Autodesk Inventor part; units mm, degrees
ref_plane "YZ Plane" through (0, 0, 0) normal (1, 0, 0) x (0, 1, 0)
ref_plane "XZ Plane" through (0, 0, 0) normal (0, 1, 0) x (-1, 0, 0)
ref_plane "XY Plane" through (0, 0, 0) normal (0, 0, 1) x (1, 0, 0)
sketch "Sketch1" plane through (0, 0, 0) normal (1, 0, 0) x (0, 1, 0)
  line L0 (0, 0) -> (55, 0)
  line L1 (55, 0) -> (55, -242)
  line L2 (55, -242) -> (0, -242)
  line L3 (0, -242) -> (0, 0)
  dimension "d0" = 55
  dimension "d1" = 242
extrude "Extrusion1" add sketch "Sketch1" along normal blind 355
sketch "Sketch3" plane through (0, 55, 0) normal (0, 1, 0) x (1, 0, 0)
  circle A0 centre (200, 120) radius 10
  point P0 (0, 0)
  point P1 (0, 0)
  dimension "d8" = 20
extrude "Extrusion3" cut sketch "Sketch3" against normal through all
sketch "Sketch4" plane through (0, 55, 0) normal (0, 1, 0) x (1, 0, 0)
  line L0 (15, 15) -> (340, 15)
  line L1 (340, 15) -> (340, 227)
  line L2 (340, 227) -> (15, 227)
  line L3 (15, 227) -> (15, 15)
  line L4 (355, 242) -> (355, 0)
  line L5 (0, 242) -> (355, 242)
  point P0 (0, 0)
  point P1 (0, 0)
  dimension "d11" = 15
  dimension "d12" = 15
extrude "Extrusion4" cut sketch "Sketch4" against normal blind 35
sketch "Sketch5" plane through (0, 0, 0) normal (0, 0, 1) x (1, 0, 0)
  circle A0 centre (161.4027, 23.0942) radius 3
  line L0 (0, 55) -> (0, 0)
  line L1 (355, 55) -> (355, 0)
  line L2 (0, 0) -> (355, 0)
  dimension "d15" = 6
  dimension "d18" = 161.4027
  dimension "d19" = 355
  dimension "d20" = 23.0942
extrude "Extrusion5" cut sketch "Sketch5" against normal through all
ref_plane "Work Plane1" through (0, 0, -121) normal (0, 0, -1) x (-1, 0, 0)
properties part number "basefresh" material "Wood (Cherry)"
Check sheet for the modelled part. Datum: model origin and axes. Units: mm. A direction names the side the tool comes from. Round coordinates to 2 decimals unless told otherwise and drop trailing zeros. Loops run counter-clockwise (first coordinate to the right, second up) from the corner with the lowest first, then second, coordinate; pieces in that order, holes last. Notation, with made-up numbers: (18.5, -28) - (41.5, -28) arc R36 ccw to (41.5, 7) - close; hole circle Ø9 at (73.25, 46). An arc over 180 degrees is marked (long way). Write item = value, one per line. Start each with the question number.
Q1. Section check D-D (z = -51.5). Record the boundary of the cut face in (x, y), plus the area to 3 significant figures.
Q2. Section check A-A (x = 200). Record the boundary of the cut face in (y, z), plus the area to 3 significant figures.
Q3. Thickness scan on L1, parallel to X at y = 24, z = -116; L2, parallel to Z at x = 200, y = 5.75; L3, parallel to Z at x = 302, y = 27.5. Record the ranges inside material, lowest first.
Q4. Release check for a two-part mould opening along Z. For faces 3 (the face through (205.38, 10.14, -128.43)), 4 (the face through (164, 55, -13)), 5 (the face through (175, 38, -15)), 6 (the face through (175, 28, -242)) record: pulls with the +Z half, pulls with the -Z half, needs draft (parallel to the pull), parting line crosses it, or undercut.
Q5. Section check B-B (z = -120). Record the boundary of the cut face in (x, y), plus the area to 3 significant figures.
Q6. Section check C-C (y = 41.5). Record the boundary of the cut face in (x, z), plus the area to 3 significant figures.
Q7. Depth check by flat-ended pin: P1, Ø12, axis at x = 229, z = -156.5, coming from the -Y side; P2, Ø5, axis at x = 161.4, y = 23.09, coming from the +Z side; P3, Ø3, axis at x = 65.5, z = -143.5, coming from the +Y side. Enter the tip coordinate at first touch or a pass-through.
Q8. Access from +Z, -Z, +X, -X, +Y, -Y to the whole of each face (thin tool, end or side, straight path). Record for faces 1 (the face through (175, 27, 0)), 2 (the face through (340, 38, -120)).
Derived:
q1.outline = (0, 0) - (355, 0) - (355, 55) - (340, 55) - (340, 20) - (15, 20) - (15, 55) - (0, 55) - close
q1.area = 8,150 mm^2
q2.outline = (0, -242) - (55, -242) - (55, -227) - (20, -227) - (20, -130) - (0, -130) - close; (0, -110) - (20, -110) - (20, -15) - (55, -15) - (55, 0) - (0, 0) - close
q2.area = 5,490 mm^2
q3.L1 = 0 to 15, 340 to 355
q3.L2 = -242 to -130, -110 to 0
q3.L3 = -242 to -227, -15 to 0
q4.face_3 = undercut
q4.face_4 = needs draft
q4.face_5 = undercut
q4.face_6 = pulls with the -Z half
q5.outline = (0, 0) - (190, 0) - (190, 20) - (15, 20) - (15, 55) - (0, 55) - close; (210, 0) - (355, 0) - (355, 55) - (340, 55) - (340, 20) - (210, 20) - close
q5.area = 7,750 mm^2
q6.outline = (0, -242) - (355, -242) - (355, 0) - (0, 0) - close; hole (15, -227) - (340, -227) - (340, -15) - (15, -15) - close
q6.area = 17,000 mm^2
q7.P1 = 0
q7.P2 = through
q7.P3 = 20
q8.face_1 = +Z, +X, -X, +Y, -Y
q8.face_2 = +Y
